Source: CAD feature listing. Evaluate the final solid. Frame: model axes, mm. Face numbers are marked on the shaded views. A direction names the side the tool comes from. Give positions to 0.01 mm unless a question says otherwise; leave off trailing zeros. Write each loop counter-clockwise with the first axis right and the second up, starting at its lowest first coordinate (ties: lowest second). Pieces come first, ordered by that corner, then holes. Notation, with made-up numbers: M 37.5,42 L 71.5,42 A12 ccw 71.5,54 Z; hole C -0.75,29.25 d11. An arc over 180 degrees is marked long. Use CSV: the item, a comma, the result in double quotes. Start each with the question number.
from build123d import *

# Parameters (mm, degrees)
SKETCH_1_W                   = 22
SKETCH_1_H                   = 1
SKETCH_2_R                   = 22
EXTRUDE_1_DEPTH              = 10
HOLE_WIZARD_M3_1_D           = 3.4
HOLE_WIZARD_M3_1_DEPTH       = 11
HOLE_WIZARD_M3_1_CBORE_D     = 4.5
HOLE_WIZARD_M3_1_CBORE_DEPTH = 6
HOLE_WIZARD_1_D              = 8
HOLE_WIZARD_1_DEPTH          = 5
HOLE_WIZARD_1_CBORE_D        = 10.16
HOLE_WIZARD_1_CBORE_DEPTH    = 3
HOLE_WIZARD_M3_2_D           = 3.4
HOLE_WIZARD_M3_2_DEPTH       = 22
HOLE_WIZARD_M3_2_CBORE_D     = 6.1
HOLE_WIZARD_M3_2_CBORE_DEPTH = 3
SKETCH_16_R                  = 2.4
EXTRUDE_2_DEPTH              = 11
SKETCH_17_R                  = 22
CUT_EXTRUDE_2_DEPTH          = 7.8
SKETCH_18_R                  = 12
EXTRUDE_3_DEPTH              = 5.5
SKETCH_19_R                  = 6
EXTRUDE_4_DEPTH              = 1
CUT_EXTRUDE_3_DEPTH          = 6
SKETCH_21_R                  = 2.2
CUT_EXTRUDE_4_DEPTH          = 3.5


with BuildPart() as part:
    # 草图1 → 旋转1 (revolve)
    with BuildSketch(Plane(origin=(0, 0, 0), x_dir=(1, 0, 0), z_dir=(0, 1, 0))):
        with Locations((11, 10.5)):
            Rectangle(SKETCH_1_W, SKETCH_1_H)
    revolve(axis=Axis((0, 0, -11), (0, 0, 1)))

    # 草图2 → 凸台-拉伸1 (add)
    with BuildSketch(Plane.XY.offset(-10)):
        Circle(SKETCH_2_R)
    extrude(amount=EXTRUDE_1_DEPTH)

    # 草图3 → 旋转2 (revolve)
    with BuildSketch(Plane(origin=(0, -14.722431864, 0), x_dir=(1, 0, 0), z_dir=(0, 1, 0))):
        Polygon((11.56, 22), (8.5, 22), (8.5, 11), (12.5, 11), (12.5, 12.5), (11.56, 12.5), align=None)
    revolve(axis=Axis((8.5, -14.722431864, -22), (0, 0, 1)))

    # 草图4 → 旋转3 (revolve)
    with BuildSketch(Plane(origin=(0, -14.722431864, 0), x_dir=(1, 0, 0), z_dir=(0, 1, 0))):
        Polygon((-5.44, 22), (-8.5, 22), (-8.5, 11), (-4.5, 11), (-4.5, 12.5), (-5.44, 12.5), align=None)
    revolve(axis=Axis((-8.5, -14.722431864, -22), (0, 0, 1)))

    # 草图5 → 旋转4 (revolve)
    with BuildSketch(Plane(origin=(0, 0, 0), x_dir=(1, 0, 0), z_dir=(0, 1, 0))):
        Polygon((-13.94, 22), (-17, 22), (-17, 11), (-13, 11), (-13, 12.5), (-13.94, 12.5), align=None)
    revolve(axis=Axis((-17, 0, -22), (0, 0, 1)))

    # 草图6 → 旋转5 (revolve)
    with BuildSketch(Plane(origin=(0, 14.722431864, 0), x_dir=(1, 0, 0), z_dir=(0, 1, 0))):
        Polygon((-5.44, 22), (-8.5, 22), (-8.5, 11), (-4.5, 11), (-4.5, 12.5), (-5.44, 12.5), align=None)
    revolve(axis=Axis((-8.5, 14.722431864, -22), (0, 0, 1)))

    # 草图7 → 旋转6 (revolve)
    with BuildSketch(Plane(origin=(0, 14.722431864, 0), x_dir=(1, 0, 0), z_dir=(0, 1, 0))):
        Polygon((11.56, 22), (8.5, 22), (8.5, 11), (12.5, 11), (12.5, 12.5), (11.56, 12.5), align=None)
    revolve(axis=Axis((8.5, 14.722431864, -22), (0, 0, 1)))

    # 草图8 → 旋转7 (revolve)
    with BuildSketch(Plane(origin=(0, 0, 0), x_dir=(1, 0, 0), z_dir=(0, 1, 0))):
        Polygon((20.06, 22), (17, 22), (17, 11), (21, 11), (21, 12.5), (20.06, 12.5), align=None)
    revolve(axis=Axis((17, 0, -22), (0, 0, 1)))

    # M3 六角头机械螺钉的柱形沉头孔1
    with Locations(Plane(origin=(0, 0, -11), x_dir=(-1, 0, 0), z_dir=(0, 0, -1))):
        with Locations((15.588457268, 9), (0, 18), (-15.588457268, 9), (-15.588457268, -9), (0, -18), (15.588457268, -9)):
            CounterBoreHole(HOLE_WIZARD_M3_1_D / 2, HOLE_WIZARD_M3_1_CBORE_D / 2, HOLE_WIZARD_M3_1_CBORE_DEPTH, depth=HOLE_WIZARD_M3_1_DEPTH)

    # 孔1
    with Locations(Plane(origin=(0, 0, -11), x_dir=(-1, 0, 0), z_dir=(0, 0, -1))):
        with Locations((0, 0)):
            CounterBoreHole(HOLE_WIZARD_1_D / 2, HOLE_WIZARD_1_CBORE_D / 2, HOLE_WIZARD_1_CBORE_DEPTH, depth=HOLE_WIZARD_1_DEPTH)

    # M3 六角头机械螺钉的柱形沉头孔2
    with Locations(Plane.XY):
        with Locations((8.5, -14.722431864), (-8.5, -14.722431864), (-17, 0), (-8.5, 14.722431864), (8.5, 14.722431864), (17, 0)):
            CounterBoreHole(HOLE_WIZARD_M3_2_D / 2, HOLE_WIZARD_M3_2_CBORE_D / 2, HOLE_WIZARD_M3_2_CBORE_DEPTH, depth=HOLE_WIZARD_M3_2_DEPTH)

    # 草图16 → 凸台-拉伸2 (add)
    with BuildSketch(Plane.XY):
        with Locations((-15.588457268, 9)):
            Circle(SKETCH_16_R)
        with Locations((0, 18)):
            Circle(SKETCH_16_R)
        with Locations((15.588457268, 9)):
            Circle(SKETCH_16_R)
        with Locations((15.588457268, -9)):
            Circle(SKETCH_16_R)
        with Locations((0, -18)):
            Circle(SKETCH_16_R)
        with Locations((-15.588457268, -9)):
            Circle(SKETCH_16_R)
    extrude(amount=-EXTRUDE_2_DEPTH)

    # 草图17 → 切除-拉伸2 (cut)
    with BuildSketch(Plane.XY):
        Circle(SKETCH_17_R)
    extrude(amount=-CUT_EXTRUDE_2_DEPTH, mode=Mode.SUBTRACT)

    # 草图18 → 凸台-拉伸3 (add)
    with BuildSketch(Plane.XY.offset(-7.8)):
        Circle(SKETCH_18_R)
    extrude(amount=EXTRUDE_3_DEPTH)

    # 草图19 → 凸台-拉伸4 (add)
    with BuildSketch(Plane.XY.offset(-2.3)):
        Circle(SKETCH_19_R)
    extrude(amount=EXTRUDE_4_DEPTH)

    # 草图20 → 切除-拉伸3 (cut)
    with BuildSketch(Plane.XY.offset(-1.3)):
        with BuildLine():
            Line((-2.55, 3.05), (2.55, 3.05))
            ThreePointArc((2.55, 3.05), (2.903553391, 2.903553391), (3.05, 2.55))
            Line((3.05, 2.55), (3.05, -2.55))
            ThreePointArc((3.05, -2.55), (2.903553391, -2.903553391), (2.55, -3.05))
            Line((2.55, -3.05), (-2.55, -3.05))
            ThreePointArc((-2.55, -3.05), (-2.903553391, -2.903553391), (-3.05, -2.55))
            Line((-3.05, -2.55), (-3.05, 2.55))
            ThreePointArc((-3.05, 2.55), (-2.903553391, 2.903553391), (-2.55, 3.05))
        make_face()
    extrude(amount=-CUT_EXTRUDE_3_DEPTH, mode=Mode.SUBTRACT)

    # 草图21 → 切除-拉伸4 (cut)
    with BuildSketch(Plane.XY.offset(-7.8)):
        with Locations((-8.5, -14.722431864)):
            Circle(SKETCH_21_R)
        with Locations((-17, 0)):
            Circle(SKETCH_21_R)
        with Locations((-8.5, 14.722431864)):
            Circle(SKETCH_21_R)
        with Locations((8.5, 14.722431864)):
            Circle(SKETCH_21_R)
        with Locations((17, 0)):
            Circle(SKETCH_21_R)
        with Locations((8.5, -14.722431864)):
            Circle(SKETCH_21_R)
    extrude(amount=-CUT_EXTRUDE_4_DEPTH, mode=Mode.SUBTRACT)


solid = part.part
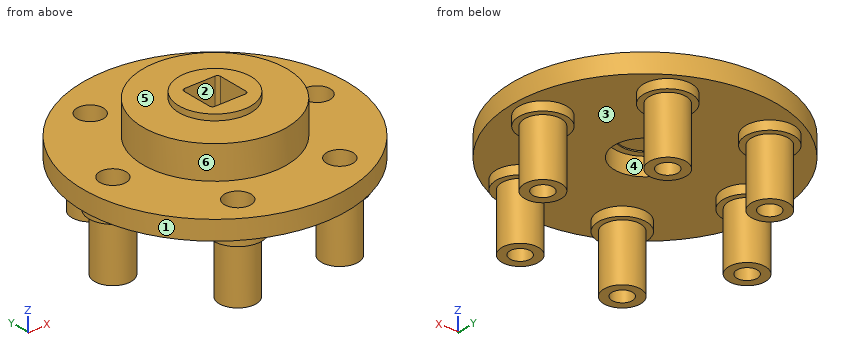
1. Section C-C on y = -15.5. Give the number of separate pieces and of enclosed holes in the cut face, then the cut area to 3 significant figures.
2. Section A-A on z = -6.5. Return loops of the section in (x, y), then the cut area to 3 significant figures.
3. First-contact query: pin 1 (2.5 mm diameter, centred on x = -8.5, y = 14.72, fed in from +Z); pin 2 (5 mm diameter, centred on x = -17, y = 0, fed in from +Z); pin 3 (6 mm diameter, centred on y = -12, z = -11, fed in from -X); pin 4 (1.5 mm diameter, centred on x = 3, y = 14.5, fed in from -Z). Flat tips, straight axial feed; report the tip coordinate or a pass-through.
4. Section B-B on x = 0. Return loops of the section in (y, z), then the cut area to 3 significant figures.
5. Pull-direction query (X, two-part tool) for the marked faces 4, 5 and 6; classes: released by +X, released by -X, zero draft, split by the parting line, or undercut.
6. Access query for the marked faces 1, 2 and 3. Directions: +Z, -Z, +X, -X, +Y, -Y. A direction counts if a zero-diameter tool reaches every point of the face in a straight line with its end or side. Return the directions, or none.
7. Line query: probe 1 along X at (y, z) = (-16, -13.5); probe 2 along Y at (x, z) = (17, -19.75); probe 3 along Y at (x, z) = (8.5, -9.95). Output: solid intervals per line, ascending.
Resolved:
1,separate pieces,"3"
1,enclosed holes,"0"
1,area,"142 mm2"
2,outline,"C 0,0 d24; hole M -3.05,-2.55 A0.5 ccw -2.55,-3.05 L 2.55,-3.05 A0.5 ccw 3.05,-2.55 L 3.05,2.55 A0.5 ccw 2.55,3.05 L -2.55,3.05 A0.5 ccw -3.05,2.55 Z"
2,area,"415 mm2"
3,pin 1,"passes through"
3,pin 2,"stops at z = -7.8"
3,pin 3,"stops at x = -20.07"
3,pin 4,"stops at z = -11"
4,outline,"M -22,-11 L -5.08,-11 L -5.08,-8 L -4,-8 L -4,-7.8 L 4,-7.8 L 4,-8 L 5.08,-8 L 5.08,-11 L 22,-11 L 22,-7.8 L 12,-7.8 L 12,-2.3 L 6,-2.3 L 6,-1.3 L 3.05,-1.3 L 3.05,-7.3 L -3.05,-7.3 L -3.05,-1.3 L -6,-1.3 L -6,-2.3 L -12,-2.3 L -12,-7.8 L -22,-7.8 Z"
4,area,"216 mm2"
5,face 4,"undercut"
5,face 5,"zero draft"
5,face 6,"split by the parting line"
6,face 1,"+Z, -Z"
6,face 2,"+Z"
6,face 3,"-Z"
7,probe 1,"x = -11.28 to -9.62, -7.38 to -5.72, 5.72 to 7.38, 9.62 to 11.28"
7,probe 2,"y = -3.06 to -1.7, 1.7 to 3.06"
7,probe 3,"y = -20.29 to -16.92, -12.52 to 12.52, 16.92 to 20.29"
